For this review, take the finished solid that the model builds, in its own axes (mm). A direction names the side the tool comes from. Coordinates: 2 decimals unless noted, no trailing zeros. Write each loop counter-clockwise with the first axis right and the second up, starting at its lowest first coordinate (ties: lowest second). Pieces come first, ordered by that corner, then holes.
1) Insertion check: P1, Ø3, axis at x = 26.5, y = 10, coming from the -Z side; P2, Ø2, axis at y = 11.5, z = 3, coming from the -X side; P3, Ø2, axis at y = 2.5, z = 3, coming from the +X side. Each pin has a flat end and moves straight along its axis. Give the tip position at first contact, or say it passes through.
2) For faces 4 (the face through (73.58, 2.12, 1.81)), 5 (the face through (1.618, 10.446, 2.328)), 6 (the face through (18.6, 8, 3)), 7 (the face through (37, 7, 0)), list the 3-axis set-ups (+Z, -Z, +X, -X, +Y, -Y) from which the entire face can be reached by the end or side of a thin tool; tool diameter is ignored.
3) We need section B-B on x = 65.5. Write out the cut boundary in (y, z), then the cut area to 3 significant figures.
4) We need section C-C on x = 11.35. Write out the cut boundary in (y, z), then the cut area to 3 significant figures.
5) We need section A-A on x = 51.7. Write out the cut boundary in (y, z).
6) Mouldability with a two-part tool opening along Y and no side actions: class faces 1 (the face through (37, 0, 3)), 2 (the face through (0, 7, 3)), 3 (the face through (25, 2.57, 2.96)) as pulls with the +Y half, pulls with the -Y half, needs draft (parallel to the pull), parting line crosses it, or undercut.
7) To check wall thickness, follow line 1 along Y through (x, z) = (11.35, 2.5); line 2 along Y through (x, z) = (73.15, 3); line 3 along X through (y, z) = (7.25, 0.75). State the ranges of each line that lie inside material, in increasing order.
8) We need section D-D on x = 24. Write out the cut boundary in (y, z).
from build123d import *

# Parameters (mm, degrees)
SKETCH1_W                                       = 75.2
SKETCH1_H                                       = 14
BOSS_EXTRUDE1_DEPTH                             = 6
SKETCH2_W                                       = 15
SKETCH2_H                                       = 7
SKETCH2_W_2                                     = 28.6
CUT_EXTRUDE1_DEPTH                              = 7
FILLET1_R                                       = 1
F_3_0_3_DIAMETER_HOLE1_D                        = 3
F_3_0_3_DIAMETER_HOLE1_DEPTH                    = 45
F_3_0_3_DIAMETER_HOLE1_TIP                      = 0.901290929
CSK_FOR_M3_FLAT_HEAD_MACHINE_SCREW1_D           = 3.4
CSK_FOR_M3_FLAT_HEAD_MACHINE_SCREW1_CSINK_D     = 6.3
CSK_FOR_M3_FLAT_HEAD_MACHINE_SCREW1_CSINK_ANGLE = 90
F_2_0_2_DIAMETER_HOLE1_D                        = 2
M3X0_5_TAPPED_HOLE1_AT_2_COUNT                  = 2
M3X0_5_TAPPED_HOLE1_AT_2_PITCH                  = 9
M3X0_5_TAPPED_HOLE2_D                           = 2.5
M3X0_5_TAPPED_HOLE2_CSINK_D                     = 3.05
M3X0_5_TAPPED_HOLE2_CSINK_ANGLE                 = 90


with BuildPart() as part:
    # Sketch1 → Boss-Extrude1 (new body)
    with BuildSketch(Plane.XY):
        with Locations((37.6, 7)):
            Rectangle(SKETCH1_W, SKETCH1_H)
    extrude(amount=BOSS_EXTRUDE1_DEPTH)

    # Sketch2 → Cut-Extrude1 (cut, through all)
    with BuildSketch(Plane.XY.offset(6)):
        with Locations((26.1, 8.5)):
            Rectangle(SKETCH2_W, SKETCH2_H)
        with Locations((55.9, 8.5)):
            Rectangle(SKETCH2_W_2, SKETCH2_H)
    extrude(amount=-CUT_EXTRUDE1_DEPTH, mode=Mode.SUBTRACT)

    # Fillet1
    fillet1_edges = [part.edges().sort_by_distance(p)[0] for p in [
        (18.6, 5, 3),
        (18.6, 12, 3),
        (33.6, 12, 3),
        (33.6, 5, 3),
        (41.6, 5, 3),
        (41.6, 12, 3),
        (70.2, 12, 3),
        (70.2, 5, 3),
    ]]
    fillet(fillet1_edges, radius=FILLET1_R)

    # Ø3.0 (3) Diameter Hole1
    with Locations(Plane.XY.offset(6)):
        with Locations((23.5, 2.5), (51.7, 2.5)):
            Hole(F_3_0_3_DIAMETER_HOLE1_D / 2, depth=F_3_0_3_DIAMETER_HOLE1_DEPTH)
            with Locations((0, 0, -(F_3_0_3_DIAMETER_HOLE1_DEPTH + F_3_0_3_DIAMETER_HOLE1_TIP / 2))):  # 118° drill point
                Cone(0, F_3_0_3_DIAMETER_HOLE1_D / 2, F_3_0_3_DIAMETER_HOLE1_TIP, mode=Mode.SUBTRACT)

    # CSK for M3 Flat Head Machine Screw1 (through all)
    with Locations(Plane(origin=(0, 0, 0), x_dir=(-1, 0, 0), z_dir=(0, 0, -1))):
        with Locations((-11.35, 11), (-15.35, 3)):
            CounterSinkHole(CSK_FOR_M3_FLAT_HEAD_MACHINE_SCREW1_D / 2, CSK_FOR_M3_FLAT_HEAD_MACHINE_SCREW1_CSINK_D / 2, counter_sink_angle=CSK_FOR_M3_FLAT_HEAD_MACHINE_SCREW1_CSINK_ANGLE)

    # Ø2.0 (2) Diameter Hole1 (through all)
    with Locations(Plane(origin=(0, 0, 0), x_dir=(-1, 0, 0), z_dir=(0, 0, -1))):
        with Locations((-15.35, 11), (-11.35, 3)):
            Hole(F_2_0_2_DIAMETER_HOLE1_D / 2)

    # Sketch12 → M3x0.5 Tapped Hole1 (revolve, cut)
    with BuildSketch(Plane(origin=(75.2, 11.5, 3), x_dir=(0, 0, -1), z_dir=(0, 1, 0))):
        Polygon((0, 0), (0, 3.751075774), (1.25, 3), (1.25, 0.275), (1.525, 0), align=None)
    m3x0_5_tapped_hole1 = revolve(axis=Axis((81.55, 11.5, 3), (-1, 0, 0)), mode=Mode.SUBTRACT)

    # M3x0.5 Tapped Hole1 at 2: M3x0.5 Tapped Hole1 ×2
    with Locations(*[(0, -i * M3X0_5_TAPPED_HOLE1_AT_2_PITCH, 0) for i in range(1, M3X0_5_TAPPED_HOLE1_AT_2_COUNT)]):
        add(m3x0_5_tapped_hole1, mode=Mode.SUBTRACT)

    # Mirror1: M3x0.5 Tapped Hole1 across plane
    add(m3x0_5_tapped_hole1.mirror(Plane(origin=(37.6, 0, 0), x_dir=(0, 0, 1), z_dir=(1, 0, 0))), mode=Mode.SUBTRACT)

    # Mirror1 copy 1 sketch → Mirror1 copy 1 (revolve, cut)
    with BuildSketch(Plane(origin=(0, 2.5, 3), x_dir=(0, 0, -1), z_dir=(0, 1, 0))):
        Polygon((0, 0), (0, -3.751075774), (1.25, -3), (1.25, -0.275), (1.525, 0), align=None)
    revolve(axis=Axis((-6.35, 2.5, 3), (-1, 0, 0)), mode=Mode.SUBTRACT)

    # M3x0.5 Tapped Hole2 (through all)
    with Locations(Plane.XY.offset(6)):
        with Locations((37.6, 9), (37.6, 5)):
            CounterSinkHole(M3X0_5_TAPPED_HOLE2_D / 2, M3X0_5_TAPPED_HOLE2_CSINK_D / 2, counter_sink_angle=M3X0_5_TAPPED_HOLE2_CSINK_ANGLE)


solid = part.part
Result:
1. P1: passes through
1. P2: stops at x = 3.15
1. P3: stops at x = 72.05
2. face 4: +X
2. face 5: -X
2. face 6: +Z, -Z
2. face 7: -Z, +X, -X, +Y, -Y
3. outline: (0, 0) - (5, 0) - (5, 6) - (0, 6) - close; (12, 0) - (14, 0) - (14, 6) - (12, 6) - close
3. area: 42.0 mm2
4. outline: (0, 0) - (2, 0) - (2, 6) - (0, 6) - close; (4, 0) - (7.85, 0) - (9.3, 1.45) - (9.3, 6) - (4, 6) - close; (12.7, 1.45) - (14, 0.15) - (14, 6) - (12.7, 6) - close
4. area: 49.5 mm2
5. outline: (0, 0) - (1, 0) - (1, 6) - (0, 6) - close; (4, 0) - (5, 0) - (5, 6) - (4, 6) - close; (12, 0) - (14, 0) - (14, 6) - (12, 6) - close
6. face 1: pulls with the -Y half
6. face 2: needs draft
6. face 3: undercut
7. line 1: y = 0 to 2, 4 to 9.3, 12.7 to 14
7. line 2: y = 0 to 1.25, 3.75 to 10.25, 12.75 to 14
7. line 3: x = 0 to 18.6, 33.6 to 41.6, 70.2 to 75.2
8. outline: (0, 0) - (1.09, 0) - (1.09, 6) - (0, 6) - close; (3.91, 0) - (5, 0) - (5, 6) - (3.91, 6) - close; (12, 0) - (14, 0) - (14, 6) - (12, 6) - close
